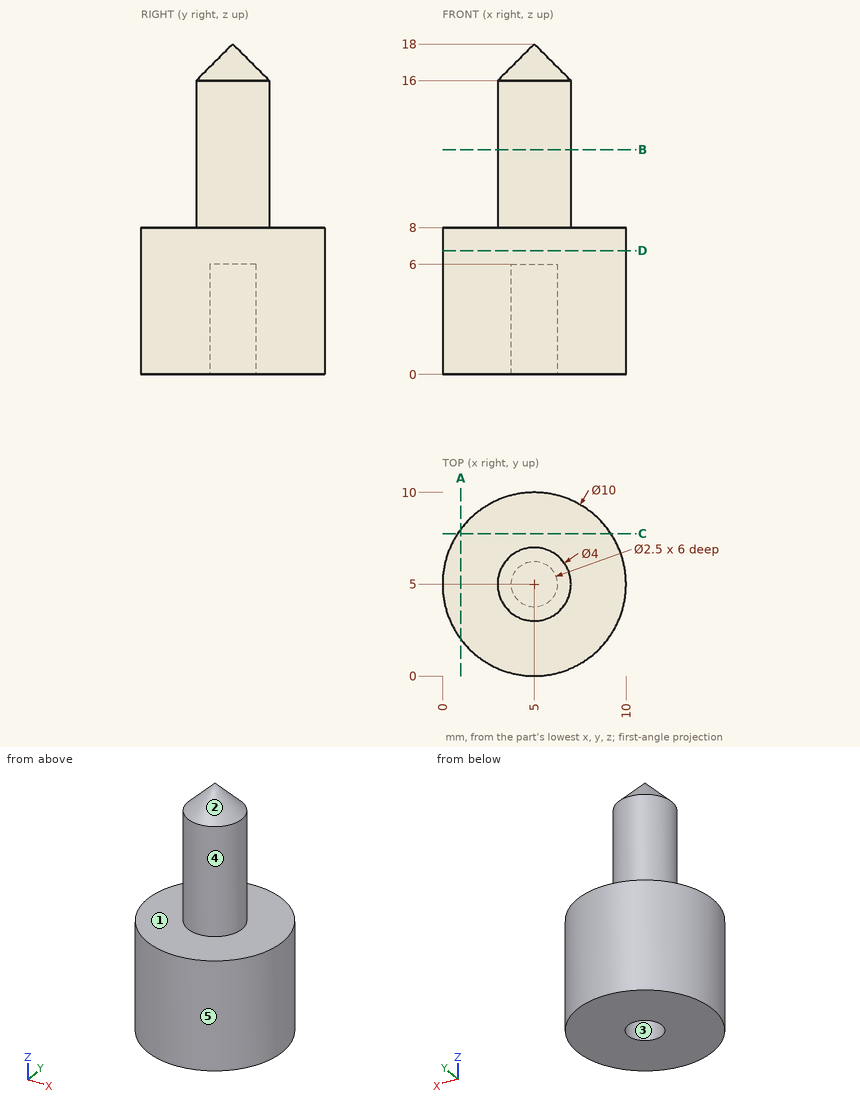
Study the drawing (mm; zero at the part's minimum x, y, z) and answer. A direction names the side the tool comes from. Give positions to 0.01 mm unless a question says otherwise; leave off trailing zeros. Write each loop counter-clockwise with the first axis right and the second up, starting at its lowest first coordinate (ties: lowest second). Pieces come first, ordered by that corner, then holes. Notation, with made-up numbers: (-37, 17) -> (-2, 17) arc R27 ccw to (-2, 33) -> close; hole circle Ø4 at (57, -12). An arc over 180 degrees is marked (long way). Write item = value, one per line. Start each with the question number.
1) The part is cut by section D-D, the plane z = 6.75. Determine the outline of the cut face in (x, y).
2) Determine the mould class of the marked faces 1, 2 and 3 for opening direction Y: +Y half, -Y half, draft (parallel to the pull), parting line (faces both ways), or undercut.
3) The part is cut by section C-C, the plane y = 7.75. Determine the outline of the cut face in (x, z).
4) Straight lines are drawn through the part: line 1 along Y through (x, z) = (5, 2); line 2 along Z through (x, y) = (0.5, 3.5); line 3 along Y through (x, z) = (4.25, 16.25). For each, find the intervals that lie inside material, in ascending order.
5) Which of the six approach directions +Z, -Z, +X, -X, +Y, -Y give full straight-line access (tool end or side, diameter ignored) to the marked faces 4 and 5?
6) The part is cut by section A-A, the plane x = 1. Determine the outline of the cut face in (y, z).
7) The part is cut by section B-B, the plane z = 12.25. Determine the outline of the cut face in (x, y).
8) Each of these flat-tipped pins is pushed along its axis until it touches: pin 1 (2 mm diameter, centred on x = 5, y = 5, fed in from -Z); pin 2 (3 mm diameter, centred on x = 7, z = 9, fed in from -Y); pin 3 (1.5 mm diameter, centred on x = 5, z = 14, fed in from -Y). Where does it stop, or does it pass through?
Solutions:
q1.outline = circle Ø10 at (5, 5)
q2.face_1 = draft
q2.face_2 = parting line
q2.face_3 = undercut
q3.outline = (0.82, 0) -> (9.18, 0) -> (9.18, 8) -> (0.82, 8) -> close
q4.line_1 = 0 to 3.75, 6.25 to 10
q4.line_2 = 0 to 8
q4.line_3 = 3.42 to 6.58
q5.face_4 = +Z
q5.face_5 = +Z, -Z
q6.outline = (2, 0) -> (8, 0) -> (8, 8) -> (2, 8) -> close
q7.outline = circle Ø4 at (5, 5)
q8.pin_1 = 6
q8.pin_2 = 0.08
q8.pin_3 = 3
